Geometry check sheet. Reference: the model listing, model coordinates, mm. Face numbers are marked on the shaded views. Round coordinates to 2 decimals unless told otherwise and drop trailing zeros. Write each loop counter-clockwise with the first axis right and the second up, starting at its lowest first coordinate (ties: lowest second). Pieces come first, ordered by that corner, then holes.
Item 1: Cross-section at B-B (y = 0). Enter the section's corners in (x, z).
Item 2: Depth check by flat-ended pin: P1, Ø4, axis at y = 17, z = 22, coming from the -X side; P2, Ø2, axis at x = 21.5, z = 11.5, coming from the -Y side; P3, Ø3, axis at y = -11, z = 12, coming from the +X side; P4, Ø1, axis at x = -26, y = 11.5, coming from the -Z side. Enter the tip coordinate at first touch or a pass-through.
Item 3: Cross-section at A-A (x = 0). Enter the section's corners in (y, z), then the cut area to 3 significant figures.
Item 4: Cross-section at D-D (x = 20). Enter the section's corners in (y, z), then the cut area to 3 significant figures.
Item 5: Draft check along X on the marked faces 1, 2 and 3. Enter one of: pulls with the +X half, pulls with the -X half, needs draft (parallel to the pull), parting line crosses it, or undercut.
Item 6: Cross-section at C-C (z = 22.5). Enter the section's corners in (x, y) (3 decimals), then the cut area to 3 significant figures.
Item 7: Scan lines: probe 1 along Y at (x, z) = (0, 11.5); probe 2 along Y at (x, z) = (-8, 1.75); probe 3 along X at (y, z) = (2, 18.5). Record each from-to range of solid material in increasing order.
from build123d import *

# Parameters (mm, degrees)
SKETCH1_R           = 44.500262214
SKETCH1_R_2         = 12.7
SKETCH1_R_3         = 3.175
BOSS_EXTRUDE1_DEPTH = 25.4
SKETCH2_R           = 3.175
CUT_EXTRUDE1_DEPTH  = 25.4


with BuildPart() as part:
    # Sketch1 → Boss-Extrude1 (new body)
    with BuildSketch(Plane.XY):
        Circle(SKETCH1_R)
        Circle(SKETCH1_R_2, mode=Mode.SUBTRACT)
        with Locations((-36.068, 0)):
            Circle(SKETCH1_R_3, mode=Mode.SUBTRACT)
        with Locations((18.034, 31.235804264)):
            Circle(SKETCH1_R_3, mode=Mode.SUBTRACT)
        with Locations((18.034, -31.235804264)):
            Circle(SKETCH1_R_3, mode=Mode.SUBTRACT)
    extrude(amount=BOSS_EXTRUDE1_DEPTH)

    # Sketch2 → Cut-Extrude1 (cut)
    with BuildSketch(Plane.XY.offset(25.4)):
        with Locations((-7.366, -31.235804264)):
            Circle(SKETCH2_R)
        with Locations((-7.366, 31.235804264)):
            Circle(SKETCH2_R)
    extrude(amount=-CUT_EXTRUDE1_DEPTH, mode=Mode.SUBTRACT)


solid = part.part
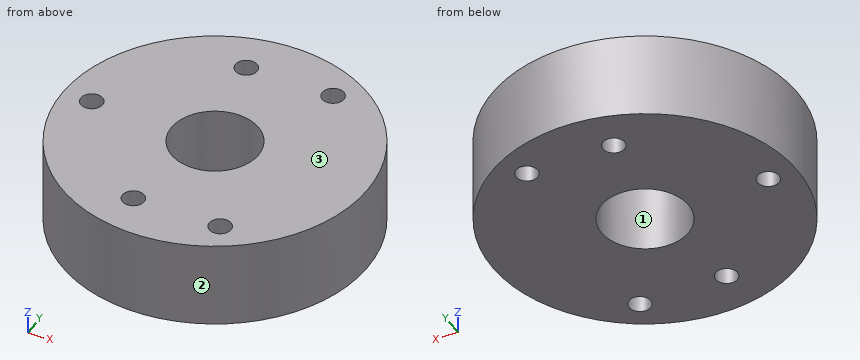
Resolved:
1. outline: (-44.5, 0) - (-39.24, 0) - (-39.24, 25.4) - (-44.5, 25.4) - close; (-32.89, 0) - (-12.7, 0) - (-12.7, 25.4) - (-32.89, 25.4) - close; (12.7, 0) - (44.5, 0) - (44.5, 25.4) - (12.7, 25.4) - close
2. P1: stops at x = -41.9
2. P2: stops at y = -39.5
2. P3: stops at x = 43.47
2. P4: stops at z = 0
3. outline: (-44.5, 0) - (-12.7, 0) - (-12.7, 25.4) - (-44.5, 25.4) - close; (12.7, 0) - (44.5, 0) - (44.5, 25.4) - (12.7, 25.4) - close
3. area: 1,620 mm2
4. outline: (-39.75, 0) - (-33.73, 0) - (-33.73, 25.4) - (-39.75, 25.4) - close; (-28.74, 0) - (28.74, 0) - (28.74, 25.4) - (-28.74, 25.4) - close; (33.73, 0) - (39.75, 0) - (39.75, 25.4) - (33.73, 25.4) - close
4. area: 1,770 mm2
5. face 1: undercut
5. face 2: parting line crosses it
5. face 3: needs draft
6. outline: circle Ø89.001 at (0, 0); hole circle Ø6.35 at (-36.068, 0); hole circle Ø25.4 at (0, 0); hole circle Ø6.35 at (-7.366, -31.236); hole circle Ø6.35 at (-7.366, 31.236); hole circle Ø6.35 at (18.034, -31.236); hole circle Ø6.35 at (18.034, 31.236)
6. area: 5,560 mm2
7. probe 1: y = -44.5 to -12.7, 12.7 to 44.5
7. probe 2: y = -43.78 to -34.35, -28.12 to -9.86, 9.86 to 28.12, 34.35 to 43.78
7. probe 3: x = -44.46 to -38.53, -33.6 to -12.54, 12.54 to 44.46
